```python
from build123d import *

# Parameters (mm, degrees)
SKETCH1_W           = 50
SKETCH1_H           = 20
BOSS_EXTRUDE1_DEPTH = 30
SKETCH2_W           = 20
SKETCH2_H           = 15
CUT_EXTRUDE1_DEPTH  = 31
SKETCH3_W           = 5
SKETCH3_H           = 20
CUT_EXTRUDE2_DEPTH  = 20
CUT_EXTRUDE3_DEPTH  = 11
CUT_EXTRUDE4_DEPTH  = 46
SKETCH7_W           = 40
SKETCH7_H           = 30
BOSS_EXTRUDE2_DEPTH = 5
SKETCH8_W           = 20
SKETCH8_H           = 15
CUT_EXTRUDE5_DEPTH  = 6
SKETCH9_W           = 40
SKETCH9_H           = 10
BOSS_EXTRUDE3_DEPTH = 10
SKETCH10_W          = 20
SKETCH10_H          = 10
CUT_EXTRUDE6_DEPTH  = 5
CUT_EXTRUDE7_DEPTH  = 16
SKETCH12_W          = 10
SKETCH12_H          = 10
BOSS_EXTRUDE4_DEPTH = 5
SKETCH13_W          = 10
SKETCH13_H          = 10
BOSS_EXTRUDE5_DEPTH = 10
SKETCH14_W          = 10
SKETCH14_H          = 10
BOSS_EXTRUDE6_DEPTH = 10
CUT_EXTRUDE8_DEPTH  = 10


with BuildPart() as part:
    # Sketch1 → Boss-Extrude1 (new body)
    with BuildSketch(Plane.XY):
        Rectangle(SKETCH1_W, SKETCH1_H)
    extrude(amount=BOSS_EXTRUDE1_DEPTH)

    # Sketch2 → Cut-Extrude1 (cut, through all)
    with BuildSketch(Plane.XY.offset(30)):
        with Locations((0, -2.5)):
            Rectangle(SKETCH2_W, SKETCH2_H)
    extrude(amount=-CUT_EXTRUDE1_DEPTH, mode=Mode.SUBTRACT)

    # Sketch3 → Cut-Extrude2 (cut)
    with BuildSketch(Plane.XY.offset(30)):
        with Locations((-22.5, 0)):
            Rectangle(SKETCH3_W, SKETCH3_H)
    extrude(amount=-CUT_EXTRUDE2_DEPTH, mode=Mode.SUBTRACT)

    # Sketch4 → Cut-Extrude3 (cut, through all)
    with BuildSketch(Plane.XY.offset(10)):
        Polygon((-20, 10), (-25, 0), (-25, 10), align=None)
    extrude(amount=-CUT_EXTRUDE3_DEPTH, mode=Mode.SUBTRACT)

    # Sketch5 → Cut-Extrude4 (cut, through all)
    with BuildSketch(Plane.ZY.offset(20)):
        Polygon((15, 10), (30, -5), (30, 10), align=None)
    extrude(amount=-CUT_EXTRUDE4_DEPTH, mode=Mode.SUBTRACT)

    # Sketch7 → Boss-Extrude2 (add)
    with BuildSketch(Plane(origin=(0, 0, 0), x_dir=(-1, 0, 0), z_dir=(0, 0, -1))):
        with Locations((-5, 5)):
            Rectangle(SKETCH7_W, SKETCH7_H)
    extrude(amount=BOSS_EXTRUDE2_DEPTH)

    # Sketch8 → Cut-Extrude5 (cut, through all)
    with BuildSketch(Plane.XY):
        with Locations((0, -2.5)):
            Rectangle(SKETCH8_W, SKETCH8_H)
    extrude(amount=-CUT_EXTRUDE5_DEPTH, mode=Mode.SUBTRACT)

    # Sketch9 → Boss-Extrude3 (add)
    with BuildSketch(Plane(origin=(0, 10, 0), x_dir=(1, 0, 0), z_dir=(0, 1, 0))):
        with Locations((5, -5)):
            Rectangle(SKETCH9_W, SKETCH9_H)
    extrude(amount=BOSS_EXTRUDE3_DEPTH)

    # Sketch10 → Cut-Extrude6 (cut)
    with BuildSketch(Plane.XY.offset(10)):
        with Locations((5, 15)):
            Rectangle(SKETCH10_W, SKETCH10_H)
    extrude(amount=-CUT_EXTRUDE6_DEPTH, mode=Mode.SUBTRACT)

    # Sketch11 → Cut-Extrude7 (cut, through all)
    with BuildSketch(Plane.XY.offset(10)):
        Polygon((-15, 20), (-10, 20), (-15, 15), align=None)
    extrude(amount=-CUT_EXTRUDE7_DEPTH, mode=Mode.SUBTRACT)

    # Sketch12 → Boss-Extrude4 (add)
    with BuildSketch(Plane.XY.offset(10)):
        with Locations((20, 15)):
            Rectangle(SKETCH12_W, SKETCH12_H)
    extrude(amount=BOSS_EXTRUDE4_DEPTH)

    # Sketch13 → Boss-Extrude5 (add)
    with BuildSketch(Plane.XY.offset(15)):
        with Locations((20, 15)):
            Rectangle(SKETCH13_W, SKETCH13_H)
    extrude(amount=BOSS_EXTRUDE5_DEPTH)

    # Sketch14 → Boss-Extrude6 (add)
    with BuildSketch(Plane.XZ.offset(-10)):
        with Locations((20, 20)):
            Rectangle(SKETCH14_W, SKETCH14_H)
    extrude(amount=BOSS_EXTRUDE6_DEPTH)

    # Sketch17 → Cut-Extrude8 (cut)
    with BuildSketch(Plane(origin=(-6.666666667, 6.666666667, 6.666666667), x_dir=(0.816496581, 0.40824829, 0.40824829), z_dir=(-0.577350269, 0.577350269, 0.577350269))):
        Polygon((26.53613888, 3.535533906), (38.783587594, -3.535533906), (26.53613888, -10.606601718), align=None)
    extrude(amount=CUT_EXTRUDE8_DEPTH, mode=Mode.SUBTRACT)


solid = part.part
```
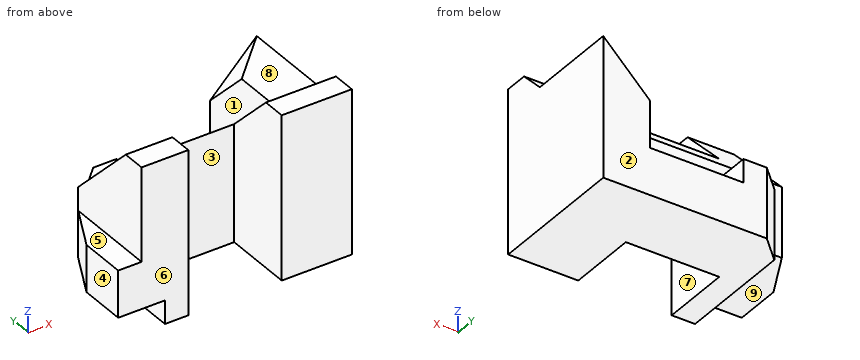
Check sheet for the modelled part. Datum: model origin and axes. Units: mm. Face numbers are marked on the shaded views. A direction names the side the tool comes from. Coordinates: 2 decimals unless noted, no trailing zeros. Write each loop counter-clockwise with the first axis right and the second up, starting at its lowest first coordinate (ties: lowest second). Pieces come first, ordered by that corner, then holes. Notation, with made-up numbers: M -11,0 L -1,0 A19 cw -1,22 Z; hole C -37,62.25 d7. An arc over 180 degrees is marked long. Use one line per item in the form item = value.
Item 1: Sectioned sample at B-B, the plane y = -2.5. Record the cut outline in (x, z).
Answer below:
outline = M -25,0 L -15,0 L -15,-5 L -10,-5 L -10,27.5 L -20,27.5 L -20,10 L -25,10 Z; M 10,-5 L 25,-5 L 25,27.5 L 10,27.5 Z
Item 2: Set-up check for the marked faces 5, 6, 7, 8 and 9: record each of +Z, -Z, +X, -X, +Y, -Y from which the full face is reachable in a straight line by a thin tool's end or side.
Answer below:
face_5 = +Z, -X, +Y, -Y
face_6 = +Z, -Z, +X, -X, -Y
face_7 = +Z, -Z, -Y
face_8 = +Z, +X, -X, +Y
face_9 = -Z, -X, +Y, -Y
Item 3: Sectioned sample at C-C, the plane y = 16. Record the cut outline in (x, z).
Answer below:
outline = M -14,-5 L 25,-5 L 25,25 L 21,25 L 15,19 L 15,5 L -5,5 L -5,10 L -14,10 Z
Item 4: Gauge pin test, flat ends, axial feed: pin 1 Ø5 at (x, y) = (-9, 16) entering from +Z; pin 2 Ø1.5 at (x, z) = (-2.5, 19.5) entering from -Y; pin 3 Ø2 at (x, z) = (16, 23.5) entering from +Y. Record the tip position at first contact, or that the pin passes through.
Answer below:
pin_1 = 10
pin_2 = 5
pin_3 = 13.91
Item 5: Sectioned sample at D-D, the plane x = -0.5. Record the cut outline in (y, z), and give its area (4 significant figures).
Answer below:
outline = M 5,-5 L 20,-5 L 20,5 L 10,5 L 10,15 L 5,20 Z
area = 212.5 mm^2
Item 6: Sectioned sample at A-A, the plane z = 21. Record the cut outline in (x, y).
Answer below:
outline = M -20,-10 L -10,-10 L -10,4 L -20,4 Z; M 10,-10 L 25,-10 L 25,20 L 21,20 L 15,14 L 15,4 L 10,4 Z
Item 7: Release check for a two-part mould opening along X. For the marked faces 1, 2, 3 and 4 record: pulls with the +X half, pulls with the -X half, needs draft (parallel to the pull), parting line crosses it, or undercut.
Answer below:
face_1 = undercut
face_2 = needs draft
face_3 = undercut
face_4 = pulls with the -X half
Item 8: Material ranges on L1, parallel to X at y = -1, z = 21; L2, parallel to X at y = 1.5, z = -3; L3, parallel to Y at x = -15.5, z = 0.5, recorded low to high. Write a range as from..to.
Answer below:
L1 = -20..-10, 10..25
L2 = -15..-10, 10..25
L3 = -10..10
